```python
from build123d import *

# Parameters (mm, degrees)
BOSS_EXTRUDE1_DEPTH = 1.5
SKETCH7_W           = 1.5
SKETCH7_H           = 24
BOSS_EXTRUDE3_DEPTH = 2


with BuildPart() as part:
    # Sketch1 → Boss-Extrude1 (new body)
    with BuildSketch(Plane.XY):
        Polygon((0, 0), (0, 297.863160558), (191.093722223, -91.025013327), (185.5038939, -100), (50, -100), (0, -50), align=None)
    extrude(amount=BOSS_EXTRUDE1_DEPTH)

    # Sketch7 → Boss-Extrude3 (add)
    with BuildSketch(Plane.ZY):
        with Locations((0.75, 235.863160558)):
            Rectangle(SKETCH7_W, SKETCH7_H)
        with Locations((0.75, 144.983352075)):
            Rectangle(SKETCH7_W, SKETCH7_H)
        with Locations((0.75, 53.983352075)):
            Rectangle(SKETCH7_W, SKETCH7_H)
    extrude(amount=BOSS_EXTRUDE3_DEPTH)


solid = part.part
```
Could you check a few things on this model? Use its own coordinates, in mm. Coordinates: 2 decimals unless noted, no trailing zeros. Write each loop counter-clockwise with the first axis right and the second up, starting at its lowest first coordinate (ties: lowest second). Pieces come first, ordered by that corner, then holes. Notation, with made-up numbers: (4, -8) -> (21, -8) arc R17 cw to (21, -4) -> close; hole circle Ø3 at (10.5, 71.25). An arc over 180 degrees is marked (long way). Write item = value, one per line. Start each with the question number.
(1) I want a section at A-A (z = 1). Please give me the cut outline in (x, y), plus the area to 3 significant figures.
(2) I want a section at C-C (y = 74). Please give me the cut outline in (x, z).
(3) I need wall thicknesses on line 1 (Y direction, x = 89.5, z = 0.9); line 2 (X direction, y = 174, z = 0.4); line 3 (Y direction, x = 145, z = 0.45). Which ranges of each line are inside material? Lowest first, please. Write a range as [from, to].
(4) I want a section at B-B (x = 152.5). Please give me the cut outline in (y, z), plus the area to 3 significant figures.
(5) Will these pins go through, and if not, where does the flat tip stop? pin 1 (0.8 mm diameter, centred on x = -1.5, z = 0.5, fed in from +Y); pin 2 (0.8 mm diameter, centred on x = -1, z = 1, fed in from -Y); pin 3 (0.8 mm diameter, centred on y = 202.5, z = 0.5, fed in from -X).
Result set:
q1.outline = (-2, 41.98) -> (0, 41.98) -> (0, -50) -> (50, -100) -> (185.5, -100) -> (191.09, -91.03) -> (0, 297.86) -> (0, 247.86) -> (-2, 247.86) -> (-2, 223.86) -> (0, 223.86) -> (0, 156.98) -> (-2, 156.98) -> (-2, 132.98) -> (0, 132.98) -> (0, 65.98) -> (-2, 65.98) -> close
q1.area = 37,700 mm2
q2.outline = (0, 0) -> (110, 0) -> (110, 1.5) -> (0, 1.5) -> close
q3.line_1 = [-100, 115.72]
q3.line_2 = [0, 60.86]
q3.line_3 = [-100, 2.78]
q4.outline = (-100, 0) -> (-12.48, 0) -> (-12.48, 1.5) -> (-100, 1.5) -> close
q4.area = 131 mm2
q5.pin_1 = 247.86
q5.pin_2 = 41.98
q5.pin_3 = 0
